Autodesk Inventor part; units mm, degrees
ref_plane "YZ Plane" through (0, 0, 0) normal (1, 0, 0) x (0, 1, 0)
ref_plane "XZ Plane" through (0, 0, 0) normal (0, 1, 0) x (-1, 0, 0)
ref_plane "XY Plane" through (0, 0, 0) normal (0, 0, 1) x (1, 0, 0)
sketch "Эскиз1" plane through (0, 0, 0) normal (0, 0, 1) x (1, 0, 0)
  circle A0 centre (0, 0) radius 2
  circle A1 centre (-39, 0) radius 2
  arc A2 (-35.1, 3.1289) -> (-42.7563, -3.3) centre (-39, 0) ccw
  arc A3 (-42.7563, -29.7) -> (-35.11, -36.1413) centre (-39, -33) ccw
  arc A4 (3.7463, -3.3114) -> (-3.9, 3.1289) centre (0, 0) ccw
  arc A5 (-3.99, -36.1413) -> (3.6663, -29.7114) centre (-0.1, -33) ccw
  arc A6 (-35.1, 3.1289) -> (-3.9, 3.1289) centre (-19.5, 15.6445) ccw
  arc A7 (3.7463, -3.3114) -> (3.6663, -29.7114) centre (18.7315, -16.5569) ccw
  arc A8 (-42.7563, -29.7) -> (-42.7563, -3.3) centre (-57.7816, -16.5) ccw
  circle A9 centre (-39, -33) radius 2
  circle A10 centre (-0.1, -33) radius 2
  arc A11 (-3.99, -36.1413) -> (-35.11, -36.1413) centre (-19.55, -48.7066) ccw
  point P0 (0, 0)
  dimension "d1" = 5
  dimension "d2" = 20
extrude "Выдавливание1" add sketch "Эскиз1" along normal blind 2
properties part number "ts_holder"
Here's how the part is built. I have some questions about the finished solid (model axes, mm). Coordinates: 2 decimals unless noted, no trailing zeros. Order: outer loops, then holes, each group sorted by start corner. A loop starts at its lowest first (then second) coordinate and runs counter-clockwise, first axis right, second up. Notation, with made-up numbers: (77, 82.5) - (120, 82.5) arc R33 cw to (120, 120.5) - close; hole circle Ø6 at (11.25, 74). An arc over 180 degrees is marked (long way). One line per question, with ' | ' between items.
(1) Will these pins go through, and if not, where does the flat tip stop? pin 1 (12 mm diameter, centred on x = -12, y = -24, fed in from -Z); pin 2 (2.5 mm diameter, centred on x = -39, y = 0, fed in from -Z).
Report:
pin 1: stops at z = 0 | pin 2: passes through
(2) Suppose I cut it at B-B on y = 0. List the corners of the cut face in (x, z) for me, and give its area (3 significant figures).
Report:
outline: (-44, 0) - (-41, 0) - (-41, 2) - (-44, 2) - close; (-37, 0) - (-31.96, 0) - (-31.96, 2) - (-37, 2) - close; (-7.04, 0) - (-2, 0) - (-2, 2) - (-7.04, 2) - close; (2, 0) - (5, 0) - (5, 2) - (2, 2) - close | area: 32.2 mm2
(3) If we mould it in two halves opening along Y, with no side actions, what happens to faces 1 (the cylindrical face through (-19.8, -28.71, 0.99)), 2 (the flat face through (-20, -16, 0)), 3 (the cylindrical face through (-42, 4, 1))? For each: pulls with the +Y half, pulls with the -Y half, needs draft (parallel to the pull), parting line crosses it, or undercut.
Report:
face 1: pulls with the -Y half | face 2: needs draft | face 3: undercut
(4) Suppose I cut it at D-D on y = -17.5. List the corners of the cut face in (x, z) for me.
Report:
outline: (-37.81, 0) - (-1.25, 0) - (-1.25, 2) - (-37.81, 2) - close
(5) If I drill on L1, parallel to Y at x = -1.5, z = 0.6; L2, parallel to X at y = 1, z = 1.1; L3, parallel to X at y = 0.5, z = 1.5, over which ranges is the centre line in solid material (lowest first)?
Report:
L1: y = -37.8 to -34.43, -31.57 to -1.32, 1.32 to 4.77 | L2: x = -43.9 to -40.73, -37.27 to -33.12, -5.88 to -1.73, 1.73 to 4.9 | L3: x = -43.97 to -40.94, -37.06 to -32.56, -6.44 to -1.94, 1.94 to 4.97
(6) Suppose I cut it at A-A on x = -39. List the corners of the cut face in (y, z) for me, and give its area (3 significant figures).
Report:
outline: (-38, 0) - (-35, 0) - (-35, 2) - (-38, 2) - close; (-31, 0) - (-23.37, 0) - (-23.37, 2) - (-31, 2) - close; (-9.63, 0) - (-2, 0) - (-2, 2) - (-9.63, 2) - close; (2, 0) - (5, 0) - (5, 2) - (2, 2) - close | area: 42.5 mm2
(7) Suppose I cut it at C-C on z = 0.7. List the corners of the cut face in (x, y) for me.
Report:
outline: (-42.76, -29.7) arc R5 ccw (long way) to (-35.11, -36.14) arc R20 cw to (-3.99, -36.14) arc R5 ccw (long way) to (3.67, -29.71) arc R20 cw to (3.75, -3.31) arc R5 ccw (long way) to (-3.9, 3.13) arc R20 cw to (-35.1, 3.13) arc R5 ccw (long way) to (-42.76, -3.3) arc R20 cw to start; hole circle Ø4 at (-39, -33); hole circle Ø4 at (-39, 0); hole circle Ø4 at (-0.1, -33); hole circle Ø4 at (0, 0)
